from build123d import *

# Parameters (mm, degrees)
EXTRUIR_L_MINA1_DEPTH = 100
CROQUIS2_R            = 6.25
CORTAR_EXTRUIR1_DEPTH = 10
CROQUIS3_R            = 7.5
CORTAR_EXTRUIR2_DEPTH = 10


with BuildPart() as part:
    # Croquis1 → Extruir-Lámina1 (new body)
    with BuildSketch(Plane.XY):
        Polygon((0, 90), (0, 0), (75, 0), (75, 10), (10, 10), (10, 90), align=None)
    extrude(amount=EXTRUIR_L_MINA1_DEPTH)

    # Croquis2 → Cortar-Extruir1 (cut)
    with BuildSketch(Plane.ZY):
        with Locations((15, 75)):
            Circle(CROQUIS2_R)
        with Locations((50, 75)):
            Circle(CROQUIS2_R)
        with Locations((85, 75)):
            Circle(CROQUIS2_R)
    extrude(amount=-CORTAR_EXTRUIR1_DEPTH, mode=Mode.SUBTRACT)

    # Croquis3 → Cortar-Extruir2 (cut)
    with BuildSketch(Plane(origin=(0, 10, 0), x_dir=(1, 0, 0), z_dir=(0, 1, 0))):
        with Locations(Location((35, -50, 0), (0, 0, 270))):
            Circle(CROQUIS3_R)
    extrude(amount=-CORTAR_EXTRUIR2_DEPTH, mode=Mode.SUBTRACT)


solid = part.part
Geometry check sheet. Reference: the model listing, model coordinates, mm. A direction names the side the tool comes from. Coordinates: 2 decimals unless noted, no trailing zeros. Order: outer loops, then holes, each group sorted by start corner. A loop starts at its lowest first (then second) coordinate and runs counter-clockwise, first axis right, second up. Notation, with made-up numbers: (3, 4.25) - (16, 4.25) arc R18 ccw to (16, 29.25) - close; hole circle Ø6 at (-21.5, 38). An arc over 180 degrees is marked (long way). Answer in a Markdown table with one row per item. Add a question column.
1) Cross-section at D-D, the plane z = 65. Record the cut outline in (x, y).
2) Cross-section at A-A, the plane z = 50. Record the cut outline in (x, y), then the cut area to 4 significant figures.
3) Gauge pin test, flat ends, axial feed: P1, Ø5, axis at y = 66.5, z = 73.5, coming from the -X side; P2, Ø2, axis at y = 45, z = 75, coming from the +X side. Record the tip position at first contact, or that the pin passes through.
4) Release check for a two-part mould opening along Y. For faces 3 (the cylindrical face through (4.93, 80.27, 88.36)), 4 (the flat face through (5, 90, 49)), 5 (the flat face through (10, 49, 49)), 6 (the cylindrical face through (4.9, 81.2, 49.2)) record: +Y half, -Y half, draft (parallel to the pull), parting line (faces both ways), or undercut.
5) Set-up check for faces 1 (the flat face through (43, 10, 49)), 2 (the flat face through (0, 46, 49)): record each of +Z, -Z, +X, -X, +Y, -Y from which the full face is reachable in a straight line by a thin tool's end or side.
6) Cross-section at C-C, the plane z = 85. Record the cut outline in (x, y).
7) Cross-section at B-B, the plane y = 75. Record the cut outline in (x, z), then the cut area to 3 significant figures.
8) Material ranges on line 1 along Y through (x, z) = (4, 50); line 2 along X through (y, z) = (56.5, 88.5), recorded low to high. Write a range as [from, to].
Check result:
| question | item | result |
|---|---|---|
| 1 | outline | (0, 0) - (75, 0) - (75, 10) - (10, 10) - (10, 90) - (0, 90) - close |
| 2 | outline | (0, 0) - (27.5, 0) - (27.5, 10) - (10, 10) - (10, 68.75) - (0, 68.75) - close; (0, 81.25) - (10, 81.25) - (10, 90) - (0, 90) - close; (42.5, 0) - (75, 0) - (75, 10) - (42.5, 10) - close |
| 2 | area | 1,275 mm² |
| 3 | P1 | stops at x = 0 |
| 3 | P2 | stops at x = 10 |
| 4 | face 3 | undercut |
| 4 | face 4 | +Y half |
| 4 | face 5 | draft |
| 4 | face 6 | undercut |
| 5 | face 1 | +Z, -Z, +X, +Y |
| 5 | face 2 | +Z, -Z, -X, +Y, -Y |
| 6 | outline | (0, 0) - (75, 0) - (75, 10) - (10, 10) - (10, 68.75) - (0, 68.75) - close; (0, 81.25) - (10, 81.25) - (10, 90) - (0, 90) - close |
| 7 | outline | (0, 0) - (10, 0) - (10, 8.75) - (0, 8.75) - close; (0, 21.25) - (10, 21.25) - (10, 43.75) - (0, 43.75) - close; (0, 56.25) - (10, 56.25) - (10, 78.75) - (0, 78.75) - close; (0, 91.25) - (10, 91.25) - (10, 100) - (0, 100) - close |
| 7 | area | 625 mm² |
| 8 | line 1 | y = [0, 68.75], [81.25, 90] |
| 8 | line 2 | x = [0, 10] |
